```python
from build123d import *

# Parameters (mm, degrees)
EXTRUDE_1_DEPTH     = 75
CUT_EXTRUDE_1_REACH = 93.984
CUT_EXTRUDE_2_DEPTH = 99.534258002


with BuildPart() as part:
    # 草图1 → 凸台-拉伸1 (new body)
    with BuildSketch(Plane.XY):
        Polygon((21, 30), (21, -29), (-21, -29), (-21, 30), (-22, 30), (-22, -30), (22, -30), (22, 30), align=None)
    extrude(amount=EXTRUDE_1_DEPTH)

    # 切除-拉伸1: up to this face of the body (flat: up to its plane)
    cut_extrude_1_end = Plane(part.part.faces().sort_by_distance((-22, 0, 37.5))[0])
    # 草图2 → 切除-拉伸1 (cut, up to the picked face)
    with BuildSketch(Plane(origin=(22, 0, 0), x_dir=(0, 0, -1), z_dir=(1, 0, 0)), mode=Mode.PRIVATE) as cut_extrude_1_sk1:
        with BuildLine():
            Line((-43.094477021, 23.429629507), (0, -29))
            Line((0, -29), (0, 30))
            Line((0, 30), (-57, 30))
            ThreePointArc((-57, 30), (-49.310179818, 28.274724746), (-43.094477021, 23.429629507))
        make_face()
    cut_extrude_1_tool1 = split(extrude(cut_extrude_1_sk1.sketch, amount=-CUT_EXTRUDE_1_REACH, mode=Mode.PRIVATE), bisect_by=cut_extrude_1_end, keep=Keep.BOTH, mode=Mode.PRIVATE)
    # 草图2 → 切除-拉伸1 (cut, up to the picked face)
    with BuildSketch(Plane(origin=(22, 0, 0), x_dir=(0, 0, -1), z_dir=(1, 0, 0)), mode=Mode.PRIVATE) as cut_extrude_1_sk2:
        with BuildLine():
            ThreePointArc((-75, 12), (-69.727922061, 24.727922061), (-57, 30))
            Line((-57, 30), (-75, 30))
            Line((-75, 30), (-75, 12))
        make_face()
    cut_extrude_1_tool2 = split(extrude(cut_extrude_1_sk2.sketch, amount=-CUT_EXTRUDE_1_REACH, mode=Mode.PRIVATE), bisect_by=cut_extrude_1_end, keep=Keep.BOTH, mode=Mode.PRIVATE)
    add(cut_extrude_1_tool1.solids().sort_by(Axis((22, 10.461352, 16.395563), (-1, 0, 0)))[0], mode=Mode.SUBTRACT)
    add(cut_extrude_1_tool2.solids().sort_by(Axis((22, 25.979377, 70.979377), (-1, 0, 0)))[0], mode=Mode.SUBTRACT)

    # 草图3 → 切除-拉伸2 (cut, through all)
    with BuildSketch(Plane.XZ.offset(30)):
        with BuildLine():
            ThreePointArc((22, 22), (15.556349186, 6.443650814), (0, 0))
            Line((0, 0), (22, 0))
            Line((22, 0), (22, 22))
        make_face()
        with BuildLine():
            ThreePointArc((0, 0), (-15.556349186, 6.443650814), (-22, 22))
            Line((-22, 22), (-22, 0))
            Line((-22, 0), (0, 0))
        make_face()
    extrude(amount=-CUT_EXTRUDE_2_DEPTH, mode=Mode.SUBTRACT)


solid = part.part
```
Geometry: final body of the model. Coordinates: model frame, mm. A direction names the side the tool comes from. Round coordinates to 2 decimals unless told otherwise and drop trailing zeros. Order: outer loops, then holes, each group sorted by start corner. A loop starts at its lowest first (then second) coordinate and runs counter-clockwise, first axis right, second up. Notation, with made-up numbers: (44.25, 73.5) -> (65.25, 73.5) arc R13 cw to (65.25, 82.5) -> close; hole circle Ø6 at (12, -38.5). An arc over 180 degrees is marked (long way). Use one line per item in the form item = value. Start each with the question number.
1. Cut plane D-D (x = 2.5). Return the cut outline in (y, z).
2. Line query: probe 1 along X at (y, z) = (13, 42); probe 2 along Y at (x, z) = (-9.5, 71). Output: solid intervals per line, ascending.
3. Reachability of faces 5 (the face through (0, -29, 37)), 6 (the face through (-21.49, 6.84, 29.46)) from +Z, -Z, +X, -X, +Y, -Y: full face, straight path, thin tool, end or side. Return the list, or none.
4. Draft query along X for faces 1 (the face through (-21, -6, 51)), 2 (the face through (-22, 0, 48)), 3 (the face through (21.51, 6.84, 29.46)), 4 (the face through (22, 0, 48)). Return one class per face: pulls with the +X half, pulls with the -X half, needs draft (parallel to the pull), parting line crosses it, or undercut.
5. Cut plane A-A (y = -16). Return the cut outline in (x, z).
6. Cut plane B-B (z = 27). Return the cut outline in (x, y), then the cut area to 3 significant figures.
7. Cut plane C-C (y = 6.5). Return the cut outline in (x, z).
8. Pin query (flat end, axial travel): pin 1 Ø6 at (x, z) = (-1, 53.5) entering from +Y. Return the tip coordinate at first contact, or that it passes through.
Solution:
q1.outline = (-30, 0.14) -> (-29, 0.14) -> (-29, 75) -> (-30, 75) -> close
q2.probe_1 = -22 to -21, 21 to 22
q2.probe_2 = -30 to -29
q3.face_5 = +Z, -Z, +Y
q3.face_6 = -Z, +X, -X, +Y
q4.face_1 = undercut
q4.face_2 = pulls with the -X half
q4.face_3 = needs draft
q4.face_4 = pulls with the +X half
q5.outline = (-22, 22) arc R22 ccw to (-21, 15.44) -> (-21, 75) -> (-22, 75) -> close; (21, 15.44) arc R22 ccw to (22, 22) -> (22, 75) -> (21, 75) -> close
q6.outline = (-22, -30) -> (22, -30) -> (22, 3.85) -> (21, 3.85) -> (21, -29) -> (-21, -29) -> (-21, 3.85) -> (-22, 3.85) -> close
q6.area = 110 mm^2
q7.outline = (-22, 29.18) -> (-21, 29.18) -> (-21, 75) -> (-22, 75) -> close; (21, 29.18) -> (22, 29.18) -> (22, 75) -> (21, 75) -> close
q8.pin_1 = -29
